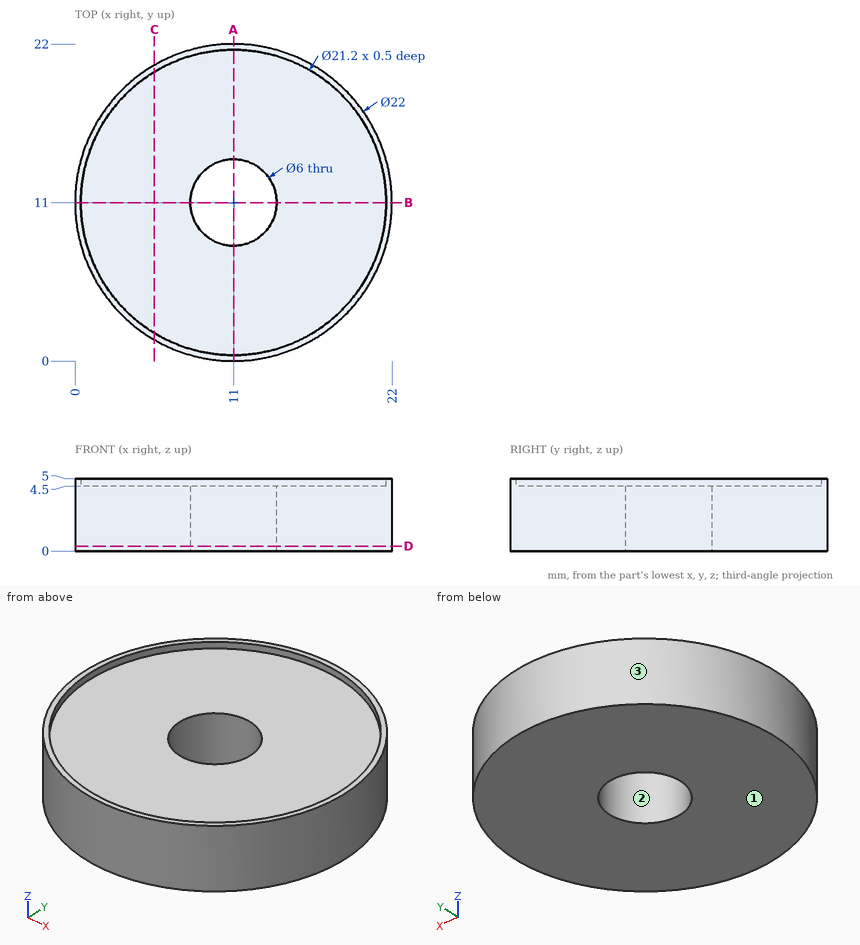
The drawing under review shows one solid part. Ordinate dimensions are in mm from its lowest x, y, z. Give positions to 0.01 mm unless a question says otherwise; leave off trailing zeros. Write each loop counter-clockwise with the first axis right and the second up, starting at its lowest first coordinate (ties: lowest second). Pieces come first, ordered by that corner, then holes. Notation, with made-up numbers: (50, 67) -> (58, 67) arc R6 cw to (58, 77) -> close; hole circle Ø11 at (28.25, 1.5). An arc over 180 degrees is marked (long way). Answer in a Markdown table with one row per item.
(1) To check wall thickness, follow probe 1 along Y at (x, z) = (11, 4.85); probe 2 along Z at (x, y) = (11, 7.75); probe 3 along Y at (x, z) = (12.75, 0.2). State the ranges of each line that lie inside material, in increasing order.
Results:
| item | result |
|---|---|
| probe 1 | 0 to 0.4, 21.6 to 22 |
| probe 2 | 0 to 4.5 |
| probe 3 | 0.14 to 8.56, 13.44 to 21.86 |
(2) Consider section A-A (x = 11). State the section outline as (y, z) points.
Results:
| item | result |
|---|---|
| outline | (0, 0) -> (8, 0) -> (8, 4.5) -> (0.4, 4.5) -> (0.4, 5) -> (0, 5) -> close; (14, 0) -> (22, 0) -> (22, 5) -> (21.6, 5) -> (21.6, 4.5) -> (14, 4.5) -> close |
(3) Clearance check with a flat-ended pin moving along its axis: pin 1 (5 mm diameter, centred on x = 15.5, y = 12.5, fed in from +Z). State where the tip first meets the part, or that it passes through.
Results:
| item | result |
|---|---|
| pin 1 | z = 4.5 |
(4) Consider section D-D (z = 0.35). State the section outline as (x, y) points, then the cut area to 3 significant figures.
Results:
| item | result |
|---|---|
| outline | circle Ø22 at (11, 11); hole circle Ø6 at (11, 11) |
| area | 352 mm2 |
(5) Consider section C-C (x = 5.5). State the section outline as (y, z) points, then the cut area to 3 significant figures.
Results:
| item | result |
|---|---|
| outline | (1.47, 0) -> (20.53, 0) -> (20.53, 5) -> (20.06, 5) -> (20.06, 4.5) -> (1.94, 4.5) -> (1.94, 5) -> (1.47, 5) -> close |
| area | 86.2 mm2 |
(6) Mouldability with a two-part tool opening along Y and no side actions: class the marked faces 1, 2 and 3 as +Y half, -Y half, draft (parallel to the pull), parting line (faces both ways), or undercut.
Results:
| item | result |
|---|---|
| face 1 | draft |
| face 2 | undercut |
| face 3 | parting line |
